Design review of the part built by this model. Coordinates are the model's own, in mm. Give positions to 0.01 mm unless a question says otherwise; leave off trailing zeros. Write each loop counter-clockwise with the first axis right and the second up, starting at its lowest first coordinate (ties: lowest second). Pieces come first, ordered by that corner, then holes. Notation, with made-up numbers: M 37.5,-1 L 67.5,-1 A27 ccw 67.5,37 Z; hole C 37,-15 d6. An arc over 180 degrees is marked long. Answer in a Markdown table with one row per item.
```python
from build123d import *

# Parameters (mm, degrees)
EXTRUDE_THIN2_DEPTH = 0.25


with BuildPart() as part:
    # Sketch1 → Extrude-Thin2 (new body, symmetric)
    with BuildSketch(Plane.XY):
        with BuildLine():
            Line((-5.85, -5.5), (-5.85, 0))
            ThreePointArc((-5.85, 0), (-5.776776695, 0.176776695), (-5.6, 0.25))
            Line((-5.6, 0.25), (5.6, 0.25))
            ThreePointArc((5.6, 0.25), (5.776776695, 0.176776695), (5.85, 0))
            Line((5.85, 0), (5.85, -5.5))
            Line((5.85, -5.5), (6.35, -5.5))
            Line((6.35, -5.5), (6.35, 0))
            ThreePointArc((6.35, 0), (6.130330086, 0.530330086), (5.6, 0.75))
            Line((5.6, 0.75), (-5.6, 0.75))
            ThreePointArc((-5.6, 0.75), (-6.130330086, 0.530330086), (-6.35, 0))
            Line((-6.35, 0), (-6.35, -5.5))
            Line((-6.35, -5.5), (-5.85, -5.5))
        make_face()
    extrude(amount=EXTRUDE_THIN2_DEPTH, both=True)


solid = part.part
```
1) Add section B-B (z = 0). Write out the cut boundary in (x, y), and give its area (3 significant figures).
Geometry says:
| item | result |
|---|---|
| outline | M -6.35,-5.5 L -5.85,-5.5 L -5.85,0 A0.25 cw -5.6,0.25 L 5.6,0.25 A0.25 cw 5.85,0 L 5.85,-5.5 L 6.35,-5.5 L 6.35,0 A0.75 ccw 5.6,0.75 L -5.6,0.75 A0.75 ccw -6.35,0 Z |
| area | 11.9 mm^2 |
2) Add section C-C (x = -1.25). Write out the cut boundary in (y, z).
Geometry says:
| item | result |
|---|---|
| outline | M 0.25,-0.25 L 0.75,-0.25 L 0.75,0.25 L 0.25,0.25 Z |
3) Add section A-A (y = -3). Write out the cut boundary in (x, z).
Geometry says:
| item | result |
|---|---|
| outline | M -6.35,-0.25 L -5.85,-0.25 L -5.85,0.25 L -6.35,0.25 Z; M 5.85,-0.25 L 6.35,-0.25 L 6.35,0.25 L 5.85,0.25 Z |
4) To check wall thickness, follow probe 1 along X at (y, z) = (-2.75, -0.2); probe 2 along Y at (x, z) = (2.25, 0.2). State the ranges of each line that lie inside material, in increasing order. Write a range as [from, to].
Geometry says:
| item | result |
|---|---|
| probe 1 | [-6.35, -5.85], [5.85, 6.35] |
| probe 2 | [0.25, 0.75] |
